from build123d import *

# Parameters (mm, degrees)
F0_R      = 12.2809
F1_DEPTH  = 18.2626
F2_R      = 2.2987
F3_DEPTH  = 4.318
F3_FACE_R = 2.2987
F4_DEPTH  = 27.7876


with BuildPart() as f1:
    # F0 (on Top) → F1 (new body)
    with BuildSketch(Plane.XY):
        Circle(F0_R)
    extrude(amount=F1_DEPTH)

    # F2 (on face) → F3 (join)
    with BuildSketch(Plane.XY.offset(18.2626)):
        Circle(F2_R)
    extrude(amount=F3_DEPTH)

    # F3_face (on face) → F4 (join)
    with BuildSketch(Plane.XY.offset(22.5806)):
        Circle(F3_FACE_R)
    extrude(amount=-F4_DEPTH)


solid = f1.part
Can you work these out from the model? Positions are in its coordinate system, mm. A direction names the side the tool comes from. Give positions to 0.01 mm unless a question says otherwise; leave off trailing zeros. Order: outer loops, then holes, each group sorted by start corner. A loop starts at its lowest first (then second) coordinate and runs counter-clockwise, first axis right, second up. Notation, with made-up numbers: M -30,67 L -24,67 A37 ccw -24,106 Z; hole C 89,-11.75 d7. An arc over 180 degrees is marked long. Use a Markdown table: item, result. Add a question column.
Item 1: For faces 1 (the cylindrical face through (2.123, -0.88, -2.567)), 2 (the cylindrical face through (-9.05, 8.3, 9)), 3 (the cylindrical face through (2.123, -0.88, 20.391)), which set-ups out of +Z, -Z, +X, -X, +Y, -Y let a thin tool reach every point of the face, with its end or its side?
Item 2: Suppose I cut it at D-D (z = 7). List the corners of the cut face in (x, y) for me.
Item 3: Will these pins go through, and if not, where does the flat tip stop? pin 1 (1 mm diameter, centred on x = -5, y = 7.5, fed in from +Z); pin 2 (3 mm diameter, centred on x = 6, y = 1.5, fed in from -Z); pin 3 (10 mm diameter, centred on x = 9.5, z = 15, fed in from -Y); pin 4 (8 mm diameter, centred on x = 5.5, y = 3, fed in from +Z).
Item 4: Suppose I cut it at A-A (y = 0). List the corners of the cut face in (x, z) for me.
Item 5: If I drill on L1, parallel to Z at x = 7.25, y = 5.75; L2, parallel to X at y = -9, z = 4.5; L3, parallel to X at y = -8, z = 6.5, over which ranges is the centre line in solid material (lowest first)? Write a range as [from, to].
Item 6: Suppose I cut it at C-C (z = 20.5). List the corners of the cut face in (x, y) for me.
Answer sheet:
| question | item | result |
|---|---|---|
| 1 | face 1 | -Z |
| 1 | face 2 | +Z, -Z |
| 1 | face 3 | +Z |
| 2 | outline | C 0,0 d24.56 |
| 3 | pin 1 | stops at z = 18.26 |
| 3 | pin 2 | stops at z = 0 |
| 3 | pin 3 | stops at y = -11.43 |
| 3 | pin 4 | stops at z = 22.58 |
| 4 | outline | M -12.28,0 L -2.3,0 L -2.3,-5.21 L 2.3,-5.21 L 2.3,0 L 12.28,0 L 12.28,18.26 L 2.3,18.26 L 2.3,22.58 L -2.3,22.58 L -2.3,18.26 L -12.28,18.26 Z |
| 5 | L1 | z = [0, 18.26] |
| 5 | L2 | x = [-8.36, 8.36] |
| 5 | L3 | x = [-9.32, 9.32] |
| 6 | outline | C 0,0 d4.6 |
